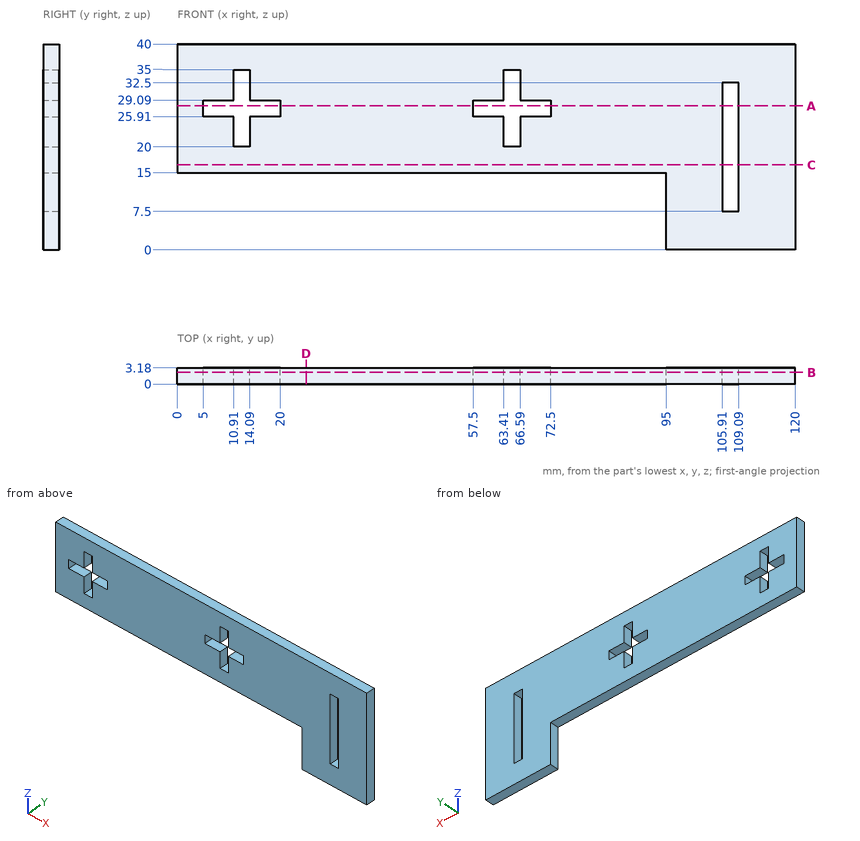
Geometry check sheet. Reference: drawing and pictorial views, mm from the part's lowest x, y, z. Coordinates: 2 decimals unless noted, no trailing zeros. Loops run counter-clockwise (first coordinate to the right, second up) from the corner with the lowest first, then second, coordinate; pieces in that order, holes last.
1) Gauge pin test, flat ends, axial feed: pin 1 (1.5 mm diameter, centred on y = 2, z = 10.5, fed in from -X); pin 2 (1.6 mm diameter, centred on x = 60.5, y = 2, fed in from -Z). Record the tip position at first contact, or that the pin passes through.
2) Sectioned sample at C-C (z = 16.5). Record the boundary of the cut face in (x, y).
3) Material ranges on probe 1 along X at (y, z) = (1.3, 24); probe 2 along Z at (x, y) = (10.5, 0.25); probe 3 along X at (y, z) = (2.5, 16.5), recorded low to high.
4) Sectioned sample at B-B (y = 2.3). Count the separate pieces of the cut face and the enclosed holes in it, and give its area (3 significant figures).
5) Sectioned sample at D-D (x = 25). Record the boundary of the cut face in (y, z).
6) Sectioned sample at A-A (z = 28). Record the boundary of the cut face in (x, y).
Check sheet entries:
1. pin 1: stops at x = 95
1. pin 2: stops at z = 15
2. outline: (0, 0) - (105.91, 0) - (105.91, 3.18) - (0, 3.18) - close; (109.09, 0) - (120, 0) - (120, 3.18) - (109.09, 3.18) - close
3. probe 1: x = 0 to 10.91, 14.09 to 63.41, 66.59 to 105.91, 109.09 to 120
3. probe 2: z = 15 to 25.91, 29.09 to 40
3. probe 3: x = 0 to 105.91, 109.09 to 120
4. separate pieces: 1
4. enclosed holes: 3
4. area: 3,120 mm2
5. outline: (0, 15) - (3.18, 15) - (3.18, 40) - (0, 40) - close
6. outline: (0, 0) - (5, 0) - (5, 3.18) - (0, 3.18) - close; (20, 0) - (57.5, 0) - (57.5, 3.18) - (20, 3.18) - close; (72.5, 0) - (105.91, 0) - (105.91, 3.18) - (72.5, 3.18) - close; (109.09, 0) - (120, 0) - (120, 3.18) - (109.09, 3.18) - close
